Part model, mm, in its own coordinate system. A direction names the side the tool comes from. Coordinates: 2 decimals unless noted, no trailing zeros. Order: outer loops, then holes, each group sorted by start corner. A loop starts at its lowest first (then second) coordinate and runs counter-clockwise, first axis right, second up.
1) Mould opens along Z. For faces 4 (the cylindrical face through (-9.474, -19.014, 10.352)), 5 (the flat face through (-10, 0, 16)), 6 (the flat face through (0, -18, 10)) say: +Z half, -Z half, draft (parallel to the pull), parting line (faces both ways), or undercut.
2) Cut at A-A (z = 3.5). List the corners of the cut face in (x, y).
3) Pin check, flat tips, straight feed: pin 1 Ø3 at (x, z) = (-8, 9) entering from +Y; pin 2 Ø1.5 at (x, y) = (3, 15) entering from +Z; pin 3 Ø3 at (x, y) = (-10, -3) entering from +Z. Stop position of each tip, or through.
4) Cut at C-C (z = 9). Give the number of separate pieces and of enclosed holes in the cut face, and give its area (4 significant figures).
5) Wall check: L1, parallel to Y at x = -7, z = 5.5; L2, parallel to Z at x = 8, y = -18.45; L3, parallel to X at y = 10.5, z = 2.25. Give the ranges that are in metal, low to high.
6) Cut at B-B (y = 0). List the corners of the cut face in (x, z).
7) Tool access for faces 1 (the flat face through (-16, 0, 9)), 2 (the cylindrical face through (-9.15, 19.01, 6.78)), 3 (the flat face through (12, 0, 8)): list every direction of +Z, -Z, +X, -X, +Y, -Y with a clear straight run to the whole face (end or side of a thin tool).
8) Cut at D-D (z = 14.25). List the corners of the cut face in (x, y), and give its area (4 significant figures).
```python
from build123d import *

# Parameters (mm, degrees)
F0_W      = 32
F0_H      = 40
F1_DEPTH  = 18
F2_W      = 28
F2_H      = 36
F3_DEPTH  = 16
F4_R      = 4
F4_R_2    = 2.5
F5_DEPTH  = 3
F6_R      = 2
F7_DEPTH  = 3
F8_R      = 4
F9_DEPTH  = 14
F10_R     = 1.5
F11_DEPTH = 8
F12_R     = 5
F13_R     = 2
F14_R     = 2


with BuildPart() as f1:
    # F0 (on Top) → F1 (new body)
    with BuildSketch(Plane.XY):
        Rectangle(F0_W, F0_H)
    extrude(amount=F1_DEPTH)

    # F2 (on face) → F3 (cut)
    with BuildSketch(Plane.XY.offset(18)):
        Rectangle(F2_W, F2_H)
    extrude(amount=-F3_DEPTH, mode=Mode.SUBTRACT)

    # F4 (on face) → F5 (cut)
    with BuildSketch(Plane(origin=(0, 20, 0), x_dir=(-1, 0, 0), z_dir=(0, 1, 0))):
        with Locations((-6, 9)):
            Circle(F4_R)
        with Locations((8, 9)):
            Circle(F4_R_2)
    extrude(amount=-F5_DEPTH, mode=Mode.SUBTRACT)

    # F6 (on face) → F7 (cut)
    with BuildSketch(Plane.XZ.offset(20)):
        with Locations((-8, 9)):
            Circle(F6_R)
        with Locations((8, 9)):
            Circle(F6_R)
    extrude(amount=-F7_DEPTH, mode=Mode.SUBTRACT)

    # F8 (on face) → F9 (join)
    with BuildSketch(Plane.XY.offset(2)):
        with Locations((-12, 0)):
            Circle(F8_R)
        with Locations((12, 0)):
            Circle(F8_R)
    extrude(amount=F9_DEPTH)

    # F10 (on face) → F11 (cut)
    with BuildSketch(Plane.XY.offset(16)):
        with Locations((-12, 0)):
            Circle(F10_R)
        with Locations((12, 0)):
            Circle(F10_R)
    extrude(amount=-F11_DEPTH, mode=Mode.SUBTRACT)

    # F12
    f12_edges = [f1.edges().sort_by_distance(p)[0] for p in [
        (14, 3.464102, 9),
        (14, -3.464102, 9),
        (-14, -3.464102, 9),
        (-14, 3.464102, 9),
    ]]
    fillet(f12_edges, radius=F12_R)

    # F13
    f13_edges = [f1.edges().sort_by_distance(p)[0] for p in [
        (-14, -18, 10),
        (14, -18, 10),
        (14, 18, 10),
        (-14, 18, 10),
    ]]
    fillet(f13_edges, radius=F13_R)

    # F14
    f14_edges = [f1.edges().sort_by_distance(p)[0] for p in [
        (16, 20, 9),
        (16, -20, 9),
        (-16, -20, 9),
        (-16, 20, 9),
    ]]
    fillet(f14_edges, radius=F14_R)


solid = f1.part
```
Geometry check:
1. face 4: undercut
1. face 5: +Z half
1. face 6: draft
2. outline: (-16, -18) arc R2 ccw to (-14, -20) - (14, -20) arc R2 ccw to (16, -18) - (16, 18) arc R2 ccw to (14, 20) - (-14, 20) arc R2 ccw to (-16, 18) - close; hole (-14, -16) arc R2 ccw to (-12, -18) - (12, -18) arc R2 ccw to (14, -16) - (14, -8.49) arc R5 ccw to (10.67, -3.77) arc R4 cw to (10.67, 3.77) arc R5 ccw to (14, 8.49) - (14, 16) arc R2 ccw to (12, 18) - (-12, 18) arc R2 ccw to (-14, 16) - (-14, 8.49) arc R5 ccw to (-10.67, 3.77) arc R4 cw to (-10.67, -3.77) arc R5 ccw to (-14, -8.49) - close
3. pin 1: stops at y = 3.12
3. pin 2: stops at z = 2
3. pin 3: stops at z = 16
4. separate pieces: 4
4. enclosed holes: 2
4. area: 312.5 mm2
5. L1: y = -20 to -18, 18 to 20
5. L2: z = 0 to 7, 11 to 18
5. L3: x = -16 to -14, 14 to 16
6. outline: (-16, 0) - (16, 0) - (16, 18) - (14, 18) - (14, 16) - (13.5, 16) - (13.5, 8) - (10.5, 8) - (10.5, 16) - (8, 16) - (8, 2) - (-8, 2) - (-8, 16) - (-10.5, 16) - (-10.5, 8) - (-13.5, 8) - (-13.5, 16) - (-14, 16) - (-14, 18) - (-16, 18) - close
7. face 1: +Z, -Z, -X, +Y, -Y
7. face 2: +Y
7. face 3: +Z
8. outline: (-16, -18) arc R2 ccw to (-14, -20) - (14, -20) arc R2 ccw to (16, -18) - (16, 18) arc R2 ccw to (14, 20) - (-14, 20) arc R2 ccw to (-16, 18) - close; hole (-14, -16) arc R2 ccw to (-12, -18) - (12, -18) arc R2 ccw to (14, -16) - (14, -8.49) arc R5 ccw to (10.67, -3.77) arc R4 cw to (10.67, 3.77) arc R5 ccw to (14, 8.49) - (14, 16) arc R2 ccw to (12, 18) - (-12, 18) arc R2 ccw to (-14, 16) - (-14, 8.49) arc R5 ccw to (-10.67, 3.77) arc R4 cw to (-10.67, -3.77) arc R5 ccw to (-14, -8.49) - close; hole circle Ø3 at (-12, 0); hole circle Ø3 at (12, 0)
8. area: 354.5 mm2
